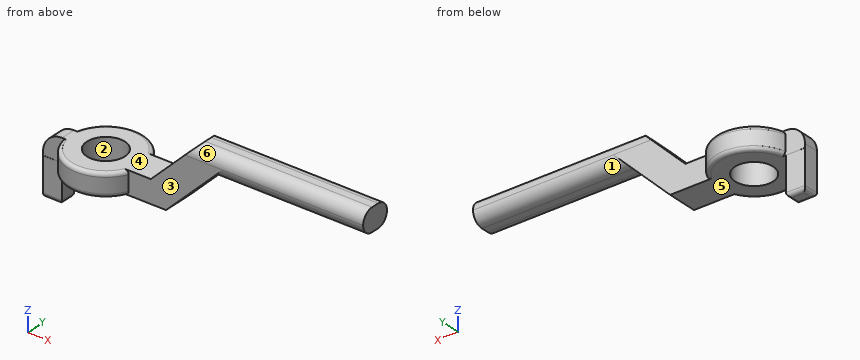
from build123d import *

# Parameters (mm, degrees)
F1_R     = 5
F2_DEPTH = 6
F4_DEPTH = 10
F5_R     = 5
F6_W     = 10
F6_H     = 8
F7_DEPTH = 6
F9_DEPTH = 6
F10_SIZE = 5.99999
F11_R    = 2.99999
F12_R    = 1
F13_R    = 1


# Not quite as in the source:
# - a fillet or chamfer is up to 0.001 mm smaller than in the source, because OpenCascade refuses the exact size


with BuildPart() as f2:
    # F1 (on offset) → F2 (new body)
    with BuildSketch(Plane.XY.offset(27)):
        with BuildLine():
            ThreePointArc((9.1651513899, -4), (9.7890631293, -2.0430964369), (10, 0))
            ThreePointArc((10, 0), (9.7890631293, 2.0430964369), (9.1651513899, 4))
            ThreePointArc((9.1651513899, 4), (-1.048861935, 9.9448423135), (-9.7979589711, 2))
            ThreePointArc((-9.7979589711, 2), (-9.9493615301, 1.0050896201), (-10, 0))
            ThreePointArc((-10, 0), (-9.9493615301, -1.0050896201), (-9.7979589711, -2))
            ThreePointArc((-9.7979589711, -2), (-1.048861935, -9.9448423135), (9.1651513899, -4))
        make_face()
        Circle(F1_R, mode=Mode.SUBTRACT)
        with BuildLine():
            Line((25, 0), (10, 0))
            ThreePointArc((10, 0), (9.7890631293, -2.0430964369), (9.1651513899, -4))
            Line((9.1651513899, -4), (25, -4))
            Line((25, -4), (25, 0))
        make_face()
        with BuildLine():
            ThreePointArc((9.1651513899, 4), (9.7890631293, 2.0430964369), (10, 0))
            Line((10, 0), (25, 0))
            Line((25, 0), (25, 4))
            Line((25, 4), (9.1651513899, 4))
        make_face()
        with BuildLine():
            ThreePointArc((-10, 0), (-9.9493615301, 1.0050896201), (-9.7979589711, 2))
            Line((-9.7979589711, 2), (-15, 2))
            Line((-15, 2), (-15, 0))
            Line((-15, 0), (-10, 0))
        make_face()
        with BuildLine():
            Line((-15, -2), (-9.7979589711, -2))
            ThreePointArc((-9.7979589711, -2), (-9.9493615301, -1.0050896201), (-10, 0))
            Line((-10, 0), (-15, 0))
            Line((-15, 0), (-15, -2))
        make_face()
    extrude(amount=F2_DEPTH)

    # F3 (on offset) → F4 (join)
    with BuildSketch(Plane.XY.offset(27)):
        Polygon((-10, -2.0203573131), (-10, 2.0309494015), (-15, 1.9722348321), (-15, -2.0203573131), align=None)
    extrude(amount=-F4_DEPTH)

    # F5
    f5_edges = [f2.edges().sort_by_distance(p)[0] for p in [
        (-15, 0, 33),
    ]]
    fillet(f5_edges, radius=F5_R)

    # F6 (on face) → F7 (join)
    with BuildSketch(Plane.XY.offset(33)):
        with Locations((20, 0)):
            Rectangle(F6_W, F6_H)
    extrude(amount=F7_DEPTH)

    # F8 (on face) → F9 (join)
    with BuildSketch(Plane.XY.offset(39)):
        Polygon((21, 4), (21, 0), (21, -4), (71, -4), (71, 4), align=None)
    extrude(amount=F9_DEPTH)

    # F10 (size 6 in the source; OpenCascade refuses exactly that, so slightly less here)
    f10_edges = [f2.edges().sort_by_distance(p)[0] for p in [
        (25, 0, 27),
        (15, 0, 39),
        (21, 0, 45),
        (25, 0, 39),
    ]]
    chamfer(f10_edges, length=F10_SIZE)

    # F11 (radius 3 in the source; OpenCascade refuses exactly that, so slightly less here)
    f11_edges = [f2.edges().sort_by_distance(p)[0] for p in [
        (48.999995, -4, 45),
        (50.999995, -4, 39),
        (50.999995, 4, 39),
        (48.999995, 4, 45),
    ]]
    fillet(f11_edges, radius=F11_R)

    # F12
    f12_edges = [f2.edges().sort_by_distance(p)[0] for p in [
        (-1.048862, -9.944842, 33),
        (-1.048862, -9.944842, 27),
        (-1.048862, 9.944842, 33),
        (-1.048862, 9.944842, 27),
    ]]
    fillet(f12_edges, radius=F12_R)

    # F13
    f13_edges = [f2.edges().sort_by_distance(p)[0] for p in [
        (-12.5, -2.020357, 17),
        (-15, -0.024061, 17),
        (-12.5, 2.001592, 17),
        (-10, 0.005296, 17),
    ]]
    fillet(f13_edges, radius=F13_R)


solid = f2.part
Geometry check sheet. Reference: the model listing, model coordinates, mm. Face numbers are marked on the shaded views. A direction names the side the tool comes from. Give positions to 0.01 mm unless a question says otherwise; leave off trailing zeros. Write each loop counter-clockwise with the first axis right and the second up, starting at its lowest first coordinate (ties: lowest second). Pieces come first, ordered by that corner, then holes. Notation, with made-up numbers: (-14.5, -12) - (3.5, -12) arc R23 ccw to (3.5, 11) - close; hole circle Ø3 at (1, 54.25). An arc over 180 degrees is marked (long way). Put each result on its own line as item: value.
1. Thickness scan on line 1 (Y direction, x = 0, z = 29.5); line 2 (X direction, y = 0.5, z = 29); line 3 (Y direction, x = 23.5, z = 39.5). Record the ranges inside material, lowest first.
Ans:
line 1: y = -10 to -5, 5 to 10
line 2: x = -14.9 to -4.97, 4.97 to 21
line 3: y = -4 to 4
2. Draft check along Y on the marked faces 1, 2 and 3. Enter one of: +Y half, -Y half, draft (parallel to the pull), parting line (faces both ways), or undercut.
Ans:
face 1: +Y half
face 2: undercut
face 3: -Y half
3. Go/stop test with flat-tipped pins: pin 1 (2 mm diameter, centred on y = -6, z = 31, fed in from +X); pin 2 (3 mm diameter, centred on y = 1, z = 22.5, fed in from +X); pin 3 (6 mm diameter, centred on x = 12, y = -5.5, fed in from +Z). Record where each tip stops, or that it passes through.
Ans:
pin 1: stops at x = 8.66
pin 2: stops at x = -10
pin 3: stops at z = 33
4. Sectioned sample at C-C, the plane z = 34.5. Enter the section's corners in (x, y), plus the area to 3 significant figures.
Ans:
outline: (16.5, -4) - (26.5, -4) - (26.5, 4) - (16.5, 4) - close
area: 80.0 mm²
5. Sectioned sample at B-B, the plane z = 25. Enter the section's corners in (x, y), plus the area to 3 significant figures.
Ans:
outline: (-15, -2.02) - (-10, -2.02) - (-10, 2.03) - (-15, 1.97) - close
area: 20.1 mm²
6. Set-up check for the marked faces 4, 5 and 6: record each of +Z, -Z, +X, -X, +Y, -Y from which the full face is reachable in a straight line by a thin tool's end or side.
Ans:
face 4: +Z, -X, +Y, -Y
face 5: -Z, +X, +Y, -Y
face 6: +Z, +X, -X, -Y
